Source: CAD feature listing. Evaluate the final solid. Frame: model axes, mm. Face numbers are marked on the shaded views. A direction names the side the tool comes from. Coordinates: 2 decimals unless noted, no trailing zeros. Order: outer loops, then holes, each group sorted by start corner. A loop starts at its lowest first (then second) coordinate and runs counter-clockwise, first axis right, second up.
Item 1: Section C-C on x = 15. Return the cut outline in (y, z), then the cut area to 3 significant figures.
Item 2: Section D-D on z = -20. Return the cut outline in (x, y), then the cut area to 3 significant figures.
Item 3: Contact query for flat-ended pins moving along their axis: P1, Ø2.5, axis at x = 0.5, y = 26, coming from the +Z side; P2, Ø1.3, axis at x = 1, y = -24, coming from the +Z side; P3, Ø3.5, axis at y = 26, z = 23, coming from the +X side; P4, Ø11, axis at x = 0, z = -30, coming from the -Y side. Output: stop coordinate, or through.
Item 4: Mould query, pull axis X, two halves, no side actions, for the marked faces 1, 2 and 3. Classes: released by +X, released by -X, zero draft, split by the parting line, or undercut.
Item 5: Reachability of the marked faces 4, 5 and 6 from +Z, -Z, +X, -X, +Y, -Y: full face, straight path, thin tool, end or side. Return the list, or none.
Item 6: Ray query, line 1 (Z direction, x = 0, y = -34.5); line 2 (Y direction, x = 0, z = 9); line 3 (X direction, y = -36, z = -30). Return the intervals inside material, ascending.
Item 7: Section A-A on y = 0. Return the cut outline in (x, z).
Item 8: Section B-B on x = 0. Return the cut outline in (y, z), then the cut area to 3 significant figures.
from build123d import *

# Parameters (mm, degrees)
SKETCH1_R           = 40
BOSS_EXTRUDE1_DEPTH = 45
SKETCH2_R           = 25
CUT_EXTRUDE1_DEPTH  = 50
SKETCH3_W           = 45
SKETCH3_H           = 45
CUT_EXTRUDE2_DEPTH  = 40
SKETCH4_W           = 10
SKETCH4_H           = 12
CUT_EXTRUDE3_DEPTH  = 40
SKETCH5_R           = 3.5
CUT_EXTRUDE4_DEPTH  = 30


with BuildPart() as part:
    # Sketch1 → Boss-Extrude1 (new, symmetric)
    with BuildSketch(Plane.XY):
        with Locations(Location((0, 0, 0), (0, 0, 180))):
            Circle(SKETCH1_R)
    extrude(amount=BOSS_EXTRUDE1_DEPTH, both=True)

    # Sketch2 → Cut-Extrude1 (cut)
    with BuildSketch(Plane.XY.offset(45)):
        Circle(SKETCH2_R)
    extrude(amount=-CUT_EXTRUDE1_DEPTH, mode=Mode.SUBTRACT)

    # Sketch3 → Cut-Extrude2 (cut)
    with BuildSketch(Plane(origin=(0, 0, -45), x_dir=(-1, 0, 0), z_dir=(0, 0, -1))):
        Rectangle(SKETCH3_W, SKETCH3_H)
    extrude(amount=-CUT_EXTRUDE2_DEPTH, mode=Mode.SUBTRACT)

    # Sketch4 → Cut-Extrude3 (cut)
    with BuildSketch(Plane.XY.offset(45)):
        with Locations((0, 21.79)):
            Rectangle(SKETCH4_W, SKETCH4_H)
    extrude(amount=-CUT_EXTRUDE3_DEPTH, mode=Mode.SUBTRACT)

    # Sketch5 → Cut-Extrude4 (cut)
    with BuildSketch(Plane(origin=(0, -40, 45), x_dir=(-1, 0, 0), z_dir=(0, -1, 0))):
        with Locations(Location((0, 15, 0), (0, 0, 180))):
            Circle(SKETCH5_R)
        with Locations(Location((0, 75, 0), (0, 0, 180))):
            Circle(SKETCH5_R)
    extrude(amount=-CUT_EXTRUDE4_DEPTH, mode=Mode.SUBTRACT)


solid = part.part
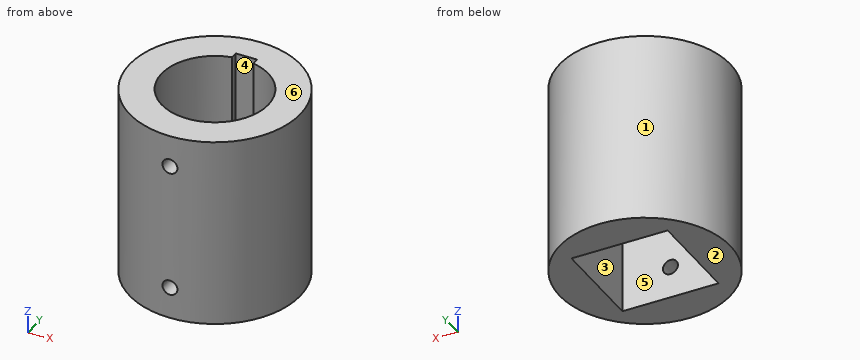
Answer list:
1. outline: (-37.08, -45) - (-22.5, -45) - (-22.5, -5) - (-20, -5) - (-20, 45) - (-37.08, 45) - close; (20, -5) - (22.5, -5) - (22.5, -45) - (37.08, -45) - (37.08, 45) - (20, 45) - close
1. area: 2,870 mm2
2. outline: circle Ø80 at (0, 0); hole (-22.5, -22.5) - (22.5, -22.5) - (22.5, 22.5) - (-22.5, 22.5) - close
2. area: 3,000 mm2
3. P1: stops at z = 5
3. P2: stops at z = -5
3. P3: stops at x = 31.81
3. P4: stops at y = -40
4. face 1: split by the parting line
4. face 2: zero draft
4. face 3: undercut
5. face 4: +Z
5. face 5: -Z
5. face 6: +Z, +X, -X, +Y, -Y
6. line 1: z = -45 to -33.5, -26.5 to 26.5, 33.5 to 45
6. line 2: y = -40 to -25, 27.79 to 40
6. line 3: x = -17.44 to -3.5, 3.5 to 17.44
7. outline: (-40, -45) - (-22.5, -45) - (-22.5, -5) - (-25, -5) - (-25, 45) - (-40, 45) - close; (22.5, -45) - (40, -45) - (40, 45) - (25, 45) - (25, -5) - (22.5, -5) - close
8. outline: (-40, -45) - (-22.5, -45) - (-22.5, -33.5) - (-40, -33.5) - close; (-40, -26.5) - (-22.5, -26.5) - (-22.5, -5) - (-25, -5) - (-25, 26.5) - (-40, 26.5) - close; (-40, 33.5) - (-25, 33.5) - (-25, 45) - (-40, 45) - close; (22.5, -45) - (40, -45) - (40, 45) - (27.79, 45) - (27.79, 5) - (25, 5) - (25, -5) - (22.5, -5) - close
8. area: 2,560 mm2
